from build123d import *
from build123d.topology import SkipClean

# Parameters (mm, degrees)
SKETCH1_R           = 80.391
BOSS_EXTRUDE1_DEPTH = 6.35
SKETCH3_R           = 4.7625
CUT_EXTRUDE2_DEPTH  = 114.867239635
THREAD1_PITCH       = 1.5875


with BuildPart() as part:
    # Sketch1 → Boss-Extrude1 (new body)
    with BuildSketch(Plane(origin=(0, 0, 0), x_dir=(1, 0, 0), z_dir=(0, 1, 0))):
        with Locations(Location((0, 0, 0), (0, 0, 270))):
            Circle(SKETCH1_R)
    extrude(amount=BOSS_EXTRUDE1_DEPTH)

    # Sketch3 → Cut-Extrude2 (cut, through all)
    with BuildSketch(Plane(origin=(0, 6.35, 0), x_dir=(1, 0, 0), z_dir=(0, 1, 0))):
        with Locations(Location((0, 0, 0), (0, 0, 270))):
            Circle(SKETCH3_R)
    extrude(amount=-CUT_EXTRUDE2_DEPTH, mode=Mode.SUBTRACT)

    # Thread1: the profile of Thread Profile1 profile screwed along a right-hand helix of 4 turns, 8 arcs to a turn; built about Z, then put on its axis
    with SkipClean():  # the faces are left unmerged after this step: merging them gives an invalid solid
        thread1_z = Axis((0, 0, 0), (0, 0, 1))
        thread1_corners = [(4.7628, 0, -0.000173205), (4.7628, 0, 1.389235701), (3.903240423, 0, 0.892968748), (3.903240423, 0, 0.496093748)]
        with BuildLine(mode=Mode.PRIVATE) as thread1_profile:
            Line(thread1_corners[0], thread1_corners[1])
            Line(thread1_corners[1], thread1_corners[2])
            Line(thread1_corners[2], thread1_corners[3])
            Line(thread1_corners[3], thread1_corners[0])
        thread1_cap = Face(thread1_profile.wire())
        thread1_turn_angles = [0, 22.5, 45, 67.5, 90, 112.5, 135, 157.5, 180, 202.5, 225, 247.5, 270, 292.5, 315, 337.5, 360]
        thread1_turn_weights = [1, 0.9238795325112867, 1, 0.9238795325112867, 1, 0.9238795325112867, 1, 0.9238795325112867, 1, 0.9238795325112867, 1, 0.9238795325112867, 1, 0.9238795325112867, 1, 0.9238795325112867, 1]
        thread1_turn_rails = [Edge.make_bspline([Vector(p[0], p[1], 0).rotate(thread1_z, thread1_turn_angles[k]) / thread1_turn_weights[k] + Vector(0, 0, p[2] + THREAD1_PITCH * thread1_turn_angles[k] / 360) for k in range(17)], [0, 0, 0, 1, 1, 2, 2, 3, 3, 4, 4, 5, 5, 6, 6, 7, 7, 8, 8, 8], 2, thread1_turn_weights) for p in thread1_corners]
        thread1_turn_sides = [Face.make_surface_from_curves(thread1_turn_rails[p[0]], thread1_turn_rails[p[1]]) for p in [(0, 1), (1, 2), (2, 3), (3, 0)]]
        thread1 = Plane(origin=(0, 6.35, 0), x_dir=(-1, 0, 0), z_dir=(0, -1, 0)) * Solid(Shell([*[p.moved(Location((0, 0, THREAD1_PITCH * i))) for i in range(4) for p in thread1_turn_sides], thread1_cap, thread1_cap.rotate(thread1_z, 1440).moved(Location((0, 0, THREAD1_PITCH * 1440 / 360)))]))
        add(thread1)


solid = part.part
Could you check a few things on this model? Use its own coordinates, in mm. Give positions to 0.01 mm unless a question says otherwise; leave off trailing zeros. Order: outer loops, then holes, each group sorted by start corner. A loop starts at its lowest first (then second) coordinate and runs counter-clockwise, first axis right, second up.
Item 1: I'm going to push flat-ended pins straight in: pin 1 (8.5 mm diameter, centred on x = 0, z = 0, fed in from -Y); pin 2 (3 mm diameter, centred on y = -0.5, z = -58.5, fed in from -X); pin 3 (8 mm diameter, centred on x = 0.5, z = 64, fed in from -Y); pin 4 (7.5 mm diameter, centred on x = 0, z = 0, fed in from +Y). Where does each tip first touch, or does it pass through?
Item 2: I need wall thicknesses on line 1 (Y direction, x = -5, z = 5); line 2 (X direction, y = 0.5, z = -2); line 3 (X direction, y = 0.75, z = -28). Which ranges of each line are inside material? Lowest first, please.
Item 3: If we section it at A-A, the plane z = 14: Write out the boundary of the cut face in (x, y).
Item 4: If we section it at B-B, the plane x = 10: Write out the boundary of the cut face in (y, z), plus the area to 3 significant figures.
Values:
1. pin 1: stops at y = -1.09
1. pin 2: stops at x = -56.6
1. pin 3: stops at y = 0
1. pin 4: passes through
2. line 1: y = 0 to 6.35
2. line 2: x = -80.37 to -3.48, 3.49 to 80.37
2. line 3: x = -75.36 to 75.36
3. outline: (-79.16, 0) - (79.16, 0) - (79.16, 6.35) - (-79.16, 6.35) - close
4. outline: (0, -79.77) - (6.35, -79.77) - (6.35, 79.77) - (0, 79.77) - close
4. area: 1,010 mm2
